from build123d import *

# Parameters (mm, degrees)
F2_DEPTH = 3
F0_R     = 3.75
F3_DEPTH = 25
F5_DEPTH = 25


with BuildPart() as f2:
    # F1 (on Top) → F2 (new body)
    with BuildSketch(Plane.XY):
        with BuildLine():
            Line((18.290832, 46.547922), (8.93864, 26.261448))
            ThreePointArc((8.93864, 26.261448), (8.657222, 23.761775), (9.923681, 21.58838))
            ThreePointArc((9.923681, 21.58838), (20.004053, 12.8209), (23.76, 0))
            ThreePointArc((23.76, 0), (19.870822, -13.026435), (9.476497, -21.788382))
            ThreePointArc((9.476497, -21.788382), (8.532906, -23.848429), (8.859869, -26.090582))
            Line((8.859869, -26.090582), (18.290832, -46.547922))
            ThreePointArc((18.290832, -46.547922), (20.006943, -48.384291), (22.479731, -48.834407))
            ThreePointArc((22.479731, -48.834407), (45.26946, -28.996787), (53.76, 0))
            ThreePointArc((53.76, 0), (45.26946, 28.996787), (22.479731, 48.834407))
            ThreePointArc((22.479731, 48.834407), (20.006943, 48.384291), (18.290832, 46.547922))
        make_face()
    extrude(amount=F2_DEPTH)

    # F0 (on Top) → F3 (cut)
    with BuildSketch(Plane.XY):
        with Locations((33, 33)):
            Circle(F0_R)
        with Locations((33, -33)):
            Circle(F0_R)
    extrude(amount=F3_DEPTH, mode=Mode.SUBTRACT)

    # F4 (on face) → F5 (cut)
    with BuildSketch(Plane.XY.offset(3)):
        with BuildLine():
            ThreePointArc((18.566805, 28.110953), (14.410164, 27.261049), (15.260068, 23.104408))
            ThreePointArc((15.260068, 23.104408), (27.689048, 0), (15.260068, -23.104408))
            ThreePointArc((15.260068, -23.104408), (14.410164, -27.261049), (18.566805, -28.110953))
            ThreePointArc((18.566805, -28.110953), (33.689048, 0), (18.566805, 28.110953))
        make_face()
    extrude(amount=-F5_DEPTH, mode=Mode.SUBTRACT)


solid = f2.part
Geometry check sheet. Reference: the model listing, model coordinates, mm. A direction names the side the tool comes from. Give positions to 0.01 mm unless a question says otherwise; leave off trailing zeros. Loops run counter-clockwise (first coordinate to the right, second up) from the corner with the lowest first, then second, coordinate; pieces in that order, holes last. Notation, with made-up numbers: (89.25, 30.25) -> (142.25, 30.25) arc R30 ccw to (142.25, 64.25) -> close; hole circle Ø9 at (54.5, -0.5). An arc over 180 degrees is marked (long way). Answer in a Markdown table with one row per item. Add a question column.
1) Material ranges on probe 1 along Y at (x, z) = (35.5, 2.2); probe 2 along Y at (x, z) = (19, 1.4); probe 3 along Y at (x, z) = (19.5, 0.45), recorded low to high. Write a range as from..to.
2) Cross-section at C-C on x = 26. Record the boundary of the cut face in (y, z), and give its area (3 significant figures).
3) Cross-section at B-B on y = 6.5. Record the boundary of the cut face in (x, z).
4) Gauge pin test, flat ends, axial feed: P1, Ø6, axis at x = 33, y = 33, coming from the -Z side; P2, Ø1.5, axis at x = 18, z = 2, coming from the +Y side. Record the tip position at first contact, or that the pin passes through.
5) Cross-section at A-A on z = 0.55. Record the boundary of the cut face in (x, y).
6) Cross-section at D-D on y = -33. Record the boundary of the cut face in (x, z), and give its area (3 significant figures).
7) Draft check along X on faces 3 (the face through (33.686, -0.466, 1.521)), 4 (the face through (8.65, 23.8, 1.48)), 5 (the face through (36, 1, 0)). Enter one of: pulls with the +X half, pulls with the -X half, needs draft (parallel to the pull), parting line crosses it, or undercut.
8) Set-up check for faces 1 (the face through (36, 1, 3)), 2 (the face through (27.686, 0.383, 1.521)): record each of +Z, -Z, +X, -X, +Y, -Y from which the full face is reachable in a straight line by a thin tool's end or side.
Outcome:
| question | item | result |
|---|---|---|
| 1 | probe 1 | y = -40.37..-35.8, -30.2..30.2, 35.8..40.37 |
| 1 | probe 2 | y = -47.6..-27.82, -20.14..-14.27, 14.27..20.14, 27.82..47.6 |
| 1 | probe 3 | y = -48.06..-27.47, -19.66..-13.58, 13.58..19.66, 27.47..48.06 |
| 2 | outline | (-47.05, 0) -> (-21.42, 0) -> (-21.42, 3) -> (-47.05, 3) -> close; (-9.52, 0) -> (9.52, 0) -> (9.52, 3) -> (-9.52, 3) -> close; (21.42, 0) -> (47.05, 0) -> (47.05, 3) -> (21.42, 3) -> close |
| 2 | area | 211 mm^2 |
| 3 | outline | (22.85, 0) -> (26.92, 0) -> (26.92, 3) -> (22.85, 3) -> close; (33.06, 0) -> (53.37, 0) -> (53.37, 3) -> (33.06, 3) -> close |
| 4 | P1 | passes through |
| 4 | P2 | stops at y = 47.31 |
| 5 | outline | (8.86, -26.09) -> (18.29, -46.55) arc R4 ccw to (22.48, -48.83) arc R53.76 ccw to (53.76, 0) arc R53.76 ccw to (22.48, 48.83) arc R4 ccw to (18.29, 46.55) -> (8.94, 26.26) arc R4 ccw to (9.92, 21.59) arc R23.76 cw to (23.76, 0) arc R23.76 cw to (9.48, -21.79) arc R4 ccw to start; hole (15.26, -23.1) arc R3 ccw to (18.57, -28.11) arc R33.69 ccw to (18.57, 28.11) arc R3 ccw to (15.26, 23.1) arc R27.69 cw to start; hole circle Ø7.5 at (33, -33); hole circle Ø7.5 at (33, 33) |
| 6 | outline | (12.05, 0) -> (29.25, 0) -> (29.25, 3) -> (12.05, 3) -> close; (36.75, 0) -> (42.44, 0) -> (42.44, 3) -> (36.75, 3) -> close |
| 6 | area | 68.7 mm^2 |
| 7 | face 3 | undercut |
| 7 | face 4 | pulls with the -X half |
| 7 | face 5 | needs draft |
| 8 | face 1 | +Z, +X, -X, +Y, -Y |
| 8 | face 2 | +Z, -Z |
